Part model, mm, in its own coordinate system. A direction names the side the tool comes from. Coordinates: 2 decimals unless noted, no trailing zeros. Order: outer loops, then holes, each group sorted by start corner. A loop starts at its lowest first (then second) coordinate and runs counter-clockwise, first axis right, second up.
```python
from build123d import *

# Parameters (mm, degrees)
SKETCH1_R               = 40
BOSS_EXTRUDE2_DEPTH     = 10
CUT_EXTRUDE1_DEPTH      = 58.445626465
CUT_EXTRUDE1_DEPTH_BACK = 58.445626465
SKETCH2_R               = 2.5
SKETCH3_R               = 37.5
CUT_EXTRUDE2_DEPTH      = 10
CUT_EXTRUDE3_REACH      = 92
CUT_EXTRUDE3_END_RADIUS = 37.5
SKETCH4_R               = 2.5
CIRPATTERN1_COUNT       = 6


with BuildPart() as part:
    # Sketch1 → Boss-Extrude2 (new, symmetric)
    with BuildSketch(Plane(origin=(0, 0, 0), x_dir=(0, 0, -1), z_dir=(1, 0, 0))):
        Circle(SKETCH1_R)
    extrude(amount=BOSS_EXTRUDE2_DEPTH, both=True)

    # Sketch2 → Cut-Extrude1 (cut, two sides: drawn at the far end of the back side and taken through both)
    with BuildSketch(Plane(origin=(0, 0, 0), x_dir=(0, 0, -1), z_dir=(1, 0, 0)).offset(-CUT_EXTRUDE1_DEPTH_BACK)):
        with Locations((14.110434629, 26.474433602)):
            Circle(SKETCH2_R)
        with Locations((29.982749365, 1.017221954)):
            Circle(SKETCH2_R)
        with Locations((15.872314736, -25.457211649)):
            Circle(SKETCH2_R)
        with Locations((-14.110434629, -26.474433602)):
            Circle(SKETCH2_R)
        with Locations((-29.982749365, -1.017221954)):
            Circle(SKETCH2_R)
        with Locations((-15.872314736, 25.457211649)):
            Circle(SKETCH2_R)
    extrude(amount=CUT_EXTRUDE1_DEPTH + CUT_EXTRUDE1_DEPTH_BACK, mode=Mode.SUBTRACT)

    # Sketch3 → Cut-Extrude2 (cut)
    with BuildSketch(Plane.ZY.offset(10)):
        Circle(SKETCH3_R)
    extrude(amount=-CUT_EXTRUDE2_DEPTH, mode=Mode.SUBTRACT)

    # Cut-Extrude3: up to this cylinder (the profile starts outside it)
    cut_extrude3_end = Plane(origin=(-5, 0, 0), z_dir=(-1, 0, 0)) * Cylinder(CUT_EXTRUDE3_END_RADIUS, 260, mode=Mode.PRIVATE)
    # Sketch4 → Cut-Extrude3 (cut, up to the surface)
    with BuildSketch(Plane(origin=(0, 40, 0), x_dir=(1, 0, 0), z_dir=(0, 1, 0)), mode=Mode.PRIVATE) as cut_extrude3_sk1:
        with Locations(Location((-5, 0, 0), (0, 0, 270))):
            Circle(SKETCH4_R)
    cut_extrude3_tool1 = extrude(cut_extrude3_sk1.sketch, amount=-CUT_EXTRUDE3_REACH, mode=Mode.PRIVATE) - cut_extrude3_end
    cut_extrude3 = cut_extrude3_tool1.solids().sort_by_distance((-5, 40, 0))[0]
    add(cut_extrude3, mode=Mode.SUBTRACT)

    # CirPattern1: Cut-Extrude3 ×6 about axis
    cirpattern1_axis = Axis((-10, 0, 0), (1, 0, 0))
    for i in range(1, CIRPATTERN1_COUNT):
        add(cut_extrude3.rotate(cirpattern1_axis, i * 360 / CIRPATTERN1_COUNT), mode=Mode.SUBTRACT)


solid = part.part
```
(1) Slice it at B-B, the plane y = 0. Give the cut face in (x, z).
(2) Slice it at C-C, the plane x = 8.5. Give the cut face in (y, z).
(3) Drop flat-ended pins along their axis: pin 1 (1 mm diameter, centred on x = 3.5, z = -2.5, fed in from +Y); pin 2 (1.5 mm diameter, centred on x = -5, y = -2, fed in from -Z); pin 3 (2 mm diameter, centred on y = 26, z = -18, fed in from -X). Give the stop position or say it passes through.
(4) Slice it at A-A, the plane z = 0. Give the cut face in (x, y), then the cut area to 3 significant figures.
(5) Probe line 1 (Y direction, x = -1.25, z = -0.5); line 2 (X direction, y = 38.9, z = 0); line 3 (X direction, y = 12, z = 19). List the from-to ranges inside material, lowest first.
(6) Slice it at D-D, the plane x = -5. Give the cut face in (y, z).
(7) Tool access for faces 1 (the face through (-2.89, 18.2, 34.21)), 2 (the face through (-5.07, 37.18, -4.88)): list every direction of +Z, -Z, +X, -X, +Y, -Y with a clear straight run to the whole face (end or side of a thin tool).
(8) Pull direction X, two halves, no side cores. Call faces 3 (the face through (4.93, 28.953, -13.785)), 4 (the face through (10, 1, 1)), 5 (the face through (-2.89, -20.53, 32.87)): +X half, -X half, draft (parallel to the pull), parting line (faces both ways), or undercut.
Here are the results:
1. outline: (-10, -40) - (10, -40) - (10, -32.27) - (0, -32.27) - (0, -37.5) - (-10, -37.5) - close; (-10, 37.5) - (0, 37.5) - (0, 32.27) - (10, 32.27) - (10, 40) - (-10, 40) - close; (0, -27.7) - (10, -27.7) - (10, 27.7) - (0, 27.7) - close
2. outline: circle Ø80 at (0, 0); hole circle Ø5 at (-26.47, 14.11); hole circle Ø5 at (-25.46, -15.87); hole circle Ø5 at (-1.02, 29.98); hole circle Ø5 at (1.02, -29.98); hole circle Ø5 at (25.46, 15.87); hole circle Ø5 at (26.47, -14.11)
3. pin 1: stops at y = 39.95
3. pin 2: stops at z = -39.98
3. pin 3: stops at x = 0
4. outline: (-10, -40) - (-7.5, -40) - (-7.5, -37.5) - (-10, -37.5) - close; (-10, 37.5) - (-7.5, 37.5) - (-7.5, 40) - (-10, 40) - close; (-2.5, -40) - (10, -40) - (10, 40) - (-2.5, 40) - (-2.5, 37.5) - (0, 37.5) - (0, -37.5) - (-2.5, -37.5) - close
4. area: 825 mm2
5. line 1: y = -40 to -37.5, 37.5 to 40
5. line 2: x = -10 to -7.5, -2.5 to 10
5. line 3: x = 0 to 10
6. outline: (-39.92, -2.5) arc R40 ccw to (-22.13, -33.32) - (-20.87, -31.15) arc R37.5 cw to (-37.42, -2.5) - close; (-39.92, 2.5) - (-37.42, 2.5) arc R37.5 cw to (-20.87, 31.15) - (-22.13, 33.32) arc R40 ccw to start; (-17.8, -35.82) arc R40 ccw to (17.8, -35.82) - (16.54, -33.65) arc R37.5 cw to (-16.54, -33.65) - close; (-17.8, 35.82) - (-16.54, 33.65) arc R37.5 cw to (16.54, 33.65) - (17.8, 35.82) arc R40 ccw to start; (20.87, -31.15) - (22.13, -33.32) arc R40 ccw to (39.92, -2.5) - (37.42, -2.5) arc R37.5 cw to start; (20.87, 31.15) arc R37.5 cw to (37.42, 2.5) - (39.92, 2.5) arc R40 ccw to (22.13, 33.32) - close
7. face 1: none
7. face 2: -X
8. face 3: draft
8. face 4: +X half
8. face 5: undercut
